Geometry check sheet. Reference: the model listing, model coordinates, mm. A direction names the side the tool comes from. Round coordinates to 2 decimals unless told otherwise and drop trailing zeros. Order: outer loops, then holes, each group sorted by start corner. A loop starts at its lowest first (then second) coordinate and runs counter-clockwise, first axis right, second up. Notation, with made-up numbers: (-38.5, 71) - (-14.5, 71) arc R23 cw to (-14.5, 109) - close; hole circle Ø7 at (39, 22.5). An arc over 180 degrees is marked (long way). Return JSON: item names as keys, results as strings. Group by question number.
Q1. Sectioned sample at A-A, the plane z = 254.06. Record the cut outline in (x, y), then the cut area to 3 significant figures.
Q2. Sectioned sample at C-C, the plane x = -1.5. Record the cut outline in (y, z).
Q3. Material ranges on line 1 along Y through (x, z) = (18.2, 254.06); line 2 along X through (y, z) = (2.5, 249.5), recorded low to high.
Q4. Tool access check on faces 4 (the flat face through (0, -16, 133)), 5 (the flat face through (0, -19, 133)). Record the directions out of +Z, -Z, +X, -X, +Y, -Y that give a thin tool (end or side, any length) a straight path to the whole face; none if there is none.
Q5. Sectioned sample at B-B, the plane y = -10. Record the cut outline in (x, z), then the cut area to 3 significant figures.
Q6. Gauge pin test, flat end, axial feed: pin 1 Ø5 at (x, y) = (-14.5, -9) entering from +Z. Record the tip position at first contact, or that the pin passes through.
Q7. Sectioned sample at D-D, the plane z = 58. Record the cut outline in (x, y), then the cut area to 3 significant figures.
Q8. Draft check along Z on faces 1 (the cylindrical face through (17.5, -9.1, 251.2)), 2 (the flat face through (-19, 0, 133)), 3 (the flat face through (17, 0, 269.06)). Enter one of: pulls with the +Z half, pulls with the -Z half, needs draft (parallel to the pull), parting line crosses it, or undercut.
```python
from build123d import *

# Parameters (mm, degrees)
SKETCH1_W               = 38
SKETCH1_H               = 38
SKETCH1_W_2             = 32
SKETCH1_H_2             = 32
BOSS_EXTRUDE1_DEPTH     = 269.06
SKETCH2_R               = 3
CUT_EXTRUDE1_DEPTH      = 1
CUT_EXTRUDE1_DEPTH_BACK = 39


with BuildPart() as part:
    # Sketch1 → Boss-Extrude1 (new body)
    with BuildSketch(Plane.XY):
        Rectangle(SKETCH1_W, SKETCH1_H)
        Rectangle(SKETCH1_W_2, SKETCH1_H_2, mode=Mode.SUBTRACT)
    extrude(amount=BOSS_EXTRUDE1_DEPTH)

    # Sketch2 → Cut-Extrude1 (cut, two sides)
    with BuildSketch(Plane(origin=(19, 0, 0), x_dir=(0, 0, -1), z_dir=(1, 0, 0))) as cut_extrude1_sk:
        with Locations((-254.06, 10)):
            Circle(SKETCH2_R)
        with Locations((-254.06, -10)):
            Circle(SKETCH2_R)
    extrude(amount=CUT_EXTRUDE1_DEPTH, mode=Mode.SUBTRACT)
    extrude(cut_extrude1_sk.sketch, amount=-CUT_EXTRUDE1_DEPTH_BACK, mode=Mode.SUBTRACT)


solid = part.part
```
Reply:
{
 "1": {"outline": "(-19, -19) - (19, -19) - (19, -13) - (16, -13) - (16, -16) - (-16, -16) - (-16, -13) - (-19, -13) - close; (-19, -7) - (-16, -7) - (-16, 7) - (-19, 7) - close; (-19, 13) - (-16, 13) - (-16, 16) - (16, 16) - (16, 13) - (19, 13) - (19, 19) - (-19, 19) - close; (16, -7) - (19, -7) - (19, 7) - (16, 7) - close", "area": "348 mm^2"},
 "2": {"outline": "(-19, 0) - (-16, 0) - (-16, 269.06) - (-19, 269.06) - close; (16, 0) - (19, 0) - (19, 269.06) - (16, 269.06) - close"},
 "3": {"line 1": "-19 to -13, -7 to 7, 13 to 19", "line 2": "-19 to -16, 16 to 19"},
 "4": {"face 4": "+Z, -Z", "face 5": "+Z, -Z, +X, -X, -Y"},
 "5": {"outline": "(-19, 0) - (-16, 0) - (-16, 251.06) - (-19, 251.06) - close; (-19, 257.06) - (-16, 257.06) - (-16, 269.06) - (-19, 269.06) - close; (16, 0) - (19, 0) - (19, 251.06) - (16, 251.06) - close; (16, 257.06) - (19, 257.06) - (19, 269.06) - (16, 269.06) - close", "area": "1,580 mm^2"},
 "6": {"pin 1": "z = 269.06"},
 "7": {"outline": "(-19, -19) - (19, -19) - (19, 19) - (-19, 19) - close; hole (-16, -16) - (16, -16) - (16, 16) - (-16, 16) - close", "area": "420 mm^2"},
 "8": {"face 1": "undercut", "face 2": "needs draft", "face 3": "pulls with the +Z half"}
}
